Source: CAD feature listing. Evaluate the final solid. Frame: model axes, mm. A direction names the side the tool comes from. Give positions to 0.01 mm unless a question says otherwise; leave off trailing zeros. Order: outer loops, then holes, each group sorted by start corner. A loop starts at its lowest first (then second) coordinate and runs counter-clockwise, first axis right, second up. Notation, with made-up numbers: M -34.75,27 L -22.75,27 A34 ccw -22.75,61 Z; hole C 20.5,74 d1. An arc over 180 degrees is marked long. Use CSV: the item, a comma, the result in double quotes. Start each with the question number.
Item 1: Access query for faces 3 (the face through (-60.97, 20.79, -5.7)), 4 (the face through (348, 44.488, -20)), 5 (the face through (-50, 22.307, -20)). Directions: +Z, -Z, +X, -X, +Y, -Y. A direction counts if a zero-diameter tool reaches every point of the face in a straight line with its end or side. Return the directions, or none.
Item 2: Ray query, probe 1 along Y at (x, z) = (364.5, -20); probe 2 along Y at (x, z) = (236.5, -10). Return the intervals inside material, ascending. Write a range as from..to.
Item 3: Section query A-A on x = 326. Return loops of the section in (y, z), and give its area (3 significant figures).
Item 4: Section query B-B on z = -25. Return loops of the section in (x, y).
Item 5: Pull-direction query (X, two-part tool) for faces 1 (the face through (203, 42, -40)), 2 (the face through (-61.28, 20.79, -33.99)); classes: +X half, -X half, draft (parallel to the pull), parting line (faces both ways), or undercut.
Item 6: First-contact query: pin 1 (10 mm diameter, centred on x = -11.5, z = -18.5, fed in from +Y); pin 2 (1.5 mm diameter, centred on x = 93, z = -28.5, fed in from -Y); pin 3 (2 mm diameter, centred on x = 250.5, z = -27.5, fed in from -Y). Flat tips, straight axial feed; report the tip coordinate or a pass-through.
Item 7: Section query C-C on y = 34.25. Return loops of the section in (x, z).
Autodesk Inventor part; units mm, degrees
ref_plane "YZ Plane" through (0, 0, 0) normal (1, 0, 0) x (0, 1, 0)
ref_plane "XZ Plane" through (0, 0, 0) normal (0, 1, 0) x (-1, 0, 0)
ref_plane "XY Plane" through (0, 0, 0) normal (0, 0, 1) x (1, 0, 0)
sketch "Szkic1" plane through (0, 0, 0) normal (0, 0, 1) x (1, 0, 0)
  line L0 (46.9852, 26.6235) -> (8.5048, 23.1186)
  line L1 (-61.9852, 19.3198) -> (-38.201, 19.3198)
  line L2 (-33.201, 19.3198) -> (-38.201, 19.3198)
  line L3 (-61.9852, 19.3198) -> (-66.9852, 19.3198)
  line L4 (46.9852, 26.6235) -> (-33.201, 19.3198)
  line L5 (46.9852, 26.6235) -> (243.11, 44.4876)
  line L6 (8.5048, 1) -> (16.799, 1)
  line L7 (8.5048, -1) -> (16.799, -1)
  line L8 (243.1277, 44.4876) -> (455.4993, 44.4876)
  line L9 (-66.9852, 19.3198) -> (-33.201, 19.3198)
  line L10 (243.2412, 47.4876) -> (455.4993, 47.4876)
  line L11 (242.9736, 47.4876) -> (46.713, 29.6112)
  line L12 (46.713, 29.6112) -> (-33.4732, 22.3074)
  line L13 (-33.4732, 22.3074) -> (-66.9852, 22.3074)
  line L14 (-66.9852, 22.3074) -> (-66.9852, 19.3198)
  line L15 (455.4993, 47.4876) -> (455.4993, 44.4876)
  line L16 (243.2412, 47.4876) -> (242.9736, 47.4876)
  line L17 (243.1277, 44.4876) -> (243.11, 44.4876)
  point P0 (0, 0)
  dimension "d1" = 3
  dimension "d2" = 3
extrude "Wyciągnięcie proste1" add sketch "Szkic1" against normal blind 40
fillet "Zaokrąglenie1" radius 20 2 edges at (-66.9852, 20.8136, 0) (-66.9852, 20.8136, -40)
properties part number "bok2"
Verdict:
1,face 3,"+Z, -X, +Y, -Y"
1,face 4,"+Z, -Z, +X, -Y"
1,face 5,"+Z, -Z, -X, +Y"
2,probe 1,"44.49..47.49"
2,probe 2,"43.89..46.9"
3,outline,"M 44.49,-40 L 47.49,-40 L 47.49,0 L 44.49,0 Z"
3,area,"120 mm2"
4,outline,"M -66.35,19.32 L -33.2,19.32 L 8.5,23.12 L 46.99,26.62 L 243.11,44.49 L 455.5,44.49 L 455.5,47.49 L 242.97,47.49 L 46.71,29.61 L -33.47,22.31 L -66.35,22.31 Z"
5,face 1,"draft"
5,face 2,"-X half"
6,pin 1,"y = 24.76"
6,pin 2,"y = 30.75"
6,pin 3,"y = 44.49"
7,outline,"M 97.64,-40 L 130.71,-40 L 130.71,0 L 97.64,0 Z"
